Source: CAD feature listing. Evaluate the final solid. Frame: model axes, mm. A direction names the side the tool comes from. Coordinates: 2 decimals unless noted, no trailing zeros. Order: outer loops, then holes, each group sorted by start corner. A loop starts at its lowest first (then second) coordinate and runs counter-clockwise, first axis right, second up. Notation, with made-up numbers: (11, -17) - (48, -17) arc R28 ccw to (48, 2) - close; hole circle Ø7 at (43, 81). An arc over 180 degrees is marked (long way). One line per question, with ' | ' between items. Start each with the question number.
(1) Section D-D (z = -24.5). Return the cut outline in (x, y), then the cut area to 3 significant figures.
(2) Line query: line 1 along Y through (x, z) = (23.5, 5.75); line 2 along Y through (x, z) = (23, 3); line 3 along Z through (x, y) = (18.5, 8.5). Output: solid intervals per line, ascending.
(3) Draft query along X for faces 4 (the flat face through (0, 0, 20)), 5 (the cylindrical face through (-20.207, -20.409, -34.51)), 6 (the cylindrical face through (-25.34, 25.19, 5.07)). Return one class per face: +X half, -X half, draft (parallel to the pull), parting line (faces both ways), or undercut.
(4) Section C-C (y = -25). Return the cut outline in (x, z).
(5) Section B-B (x = -22.5). Return the cut outline in (y, z), then the cut area to 3 significant figures.
(6) Section A-A (z = 6). Return the cut outline in (x, y), then the cut area to 3 significant figures.
(7) Contact query for flat-ended pins moving along their axis: P1, Ø4, axis at x = 22, y = -23, coming from the -Z side; P2, Ø8, axis at x = -4, y = -7.5, coming from the +Z side; P3, Ø4.5, axis at x = -23.5, y = 23.5, coming from the +Z side. Output: stop coordinate, or through.
(8) Access query for faces 1 (the flat face through (24.4, 26, 0)), 2 (the cylindrical face through (-3.233, 1.341, 14.93)), 3 (the flat face through (-26, -24.4, 0)). Directions: +Z, -Z, +X, -X, +Y, -Y. A direction counts if a zero-diameter tool reaches every point of the face in a straight line with its end or side. Return the directions, or none.
from build123d import *

# Parameters (mm, degrees)
SKETCH1_W           = 59
SKETCH1_H           = 59
BOSS_EXTRUDE1_DEPTH = 10
SKETCH2_R           = 2.5
CUT_EXTRUDE2_DEPTH  = 43.901048938
SKETCH4_R           = 3.5
BOSS_EXTRUDE2_DEPTH = 10
BOSS_EXTRUDE3_DEPTH = 70


with BuildPart() as part:
    # Sketch1 → Boss-Extrude1 (new body)
    with BuildSketch(Plane.XY):
        Rectangle(SKETCH1_W, SKETCH1_H)
    extrude(amount=BOSS_EXTRUDE1_DEPTH)

    # Sketch2 → Cut-Extrude2 (cut, through all)
    with BuildSketch(Plane.XY.offset(10)):
        with Locations((23.5, 23.5)):
            Circle(SKETCH2_R)
        with Locations((23.5, -23.5)):
            Circle(SKETCH2_R)
        with Locations((-23.5, -23.5)):
            Circle(SKETCH2_R)
        with Locations((-23.5, 23.5)):
            Circle(SKETCH2_R)
    extrude(amount=-CUT_EXTRUDE2_DEPTH, mode=Mode.SUBTRACT)

    # Sketch4 → Boss-Extrude2 (add)
    with BuildSketch(Plane.XY.offset(10)):
        with Locations(Location((0, 0, 0), (0, 0, 180))):
            Circle(SKETCH4_R)
    extrude(amount=BOSS_EXTRUDE2_DEPTH)

    # Sketch5 → Boss-Extrude3 (add)
    with BuildSketch(Plane(origin=(0, 0, 0), x_dir=(-1, 0, 0), z_dir=(0, 0, -1))):
        with BuildLine():
            Line((-29.5, 16.5), (-29.5, -16.5))
            ThreePointArc((-29.5, -16.5), (-20.307611845, -20.307611845), (-16.5, -29.5))
            Line((-16.5, -29.5), (16.5, -29.5))
            ThreePointArc((16.5, -29.5), (20.307611845, -20.307611845), (29.5, -16.5))
            Line((29.5, -16.5), (29.5, 16.5))
            ThreePointArc((29.5, 16.5), (20.307611845, 20.307611845), (16.5, 29.5))
            Line((16.5, 29.5), (-16.5, 29.5))
            ThreePointArc((-16.5, 29.5), (-20.307611845, 20.307611845), (-29.5, 16.5))
        make_face()
    extrude(amount=BOSS_EXTRUDE3_DEPTH)


solid = part.part
Response values:
1) outline: (-29.5, -16.5) arc R13 cw to (-16.5, -29.5) - (16.5, -29.5) arc R13 cw to (29.5, -16.5) - (29.5, 16.5) arc R13 cw to (16.5, 29.5) - (-16.5, 29.5) arc R13 cw to (-29.5, 16.5) - close | area: 2,950 mm²
2) line 1: y = -29.5 to -26, -21 to 21, 26 to 29.5 | line 2: y = -29.5 to -25.95, -21.05 to 21.05, 25.95 to 29.5 | line 3: z = -70 to 10
3) face 4: draft | face 5: -X half | face 6: undercut
4) outline: (-29.5, 0) - (-25.5, 0) - (-25.5, 10) - (-29.5, 10) - close; (-21.5, 0) - (-17.3, 0) - (-17.3, -70) - (17.3, -70) - (17.3, 0) - (21.5, 0) - (21.5, 10) - (-21.5, 10) - close; (25.5, 0) - (29.5, 0) - (29.5, 10) - (25.5, 10) - close
5) outline: (-29.5, 0) - (-25.79, 0) - (-25.79, 10) - (-29.5, 10) - close; (-21.21, 0) - (-18.55, 0) - (-18.55, -70) - (18.55, -70) - (18.55, 0) - (21.21, 0) - (21.21, 10) - (-21.21, 10) - close; (25.79, 0) - (29.5, 0) - (29.5, 10) - (25.79, 10) - close | area: 3,090 mm²
6) outline: (-29.5, -29.5) - (29.5, -29.5) - (29.5, 29.5) - (-29.5, 29.5) - close; hole circle Ø5 at (-23.5, -23.5); hole circle Ø5 at (-23.5, 23.5); hole circle Ø5 at (23.5, -23.5); hole circle Ø5 at (23.5, 23.5) | area: 3,400 mm²
7) P1: stops at z = 0 | P2: stops at z = 10 | P3: passes through
8) face 1: -Z, +X, +Y | face 2: +Z | face 3: -Z, -X, -Y
